from build123d import *

# Parameters (mm, degrees)
SKETCH_1_R          = 13
SKETCH_1_R_2        = 2.6
SKETCH_1_R_3        = 1.4
EXTRUDE_1_DEPTH     = 4
SKETCH_1_3_R        = 13
SKETCH_1_3_R_2      = 2.6
EXTRUDE_2_DEPTH     = 12
EXTRUDE_START       = 11
SKETCH_1_6_R        = 14
SKETCH_1_6_R_2      = 13
EXTRUDE_3_DEPTH     = 1
CUT_EXTRUDE_1_DEPTH = 5
SKETCH_6_R          = 7.6
SKETCH_6_W          = 3
SKETCH_6_H          = 3
CUT_EXTRUDE_5_DEPTH = 5
SKETCH_5_R          = 5
CUT_EXTRUDE_6_DEPTH = 2
FILLET_1_R          = 12
SKETCH_7_R          = 20
SKETCH_7_R_2        = 13
EXTRUDE_5_DEPTH     = 11


with BuildPart() as part:
    # 草图1 → 凸台-拉伸1 (new body)
    # profile 1 of 3: a face of its own
    with BuildSketch(Plane.XY):
        Circle(SKETCH_1_R)
        Circle(SKETCH_1_R_2, mode=Mode.SUBTRACT)
    # profile 2 of 3: a face of its own
    with BuildSketch(Plane.XY):
        with BuildLine():
            Line((-1.6, -2.049390153), (-1.6, 2.049390153))
            ThreePointArc((-1.6, 2.049390153), (-2.6, 0), (-1.6, -2.049390153))
        make_face()
    # profile 3 of 3: a face of its own
    with BuildSketch(Plane.XY):
        with BuildLine():
            ThreePointArc((2.6, 0), (1.140175425, 2.336664289), (-1.6, 2.049390153))
            Line((-1.6, 2.049390153), (-1.6, -2.049390153))
            ThreePointArc((-1.6, -2.049390153), (1.140175425, -2.336664289), (2.6, 0))
        make_face()
        Circle(SKETCH_1_R_3, mode=Mode.SUBTRACT)
    extrude(amount=EXTRUDE_1_DEPTH)

    # 草图1<3> → 凸台-拉伸2 (add)
    # profile 1 of 2: a face of its own
    with BuildSketch(Plane.XY):
        Circle(SKETCH_1_3_R)
        Circle(SKETCH_1_3_R_2, mode=Mode.SUBTRACT)
    # profile 2 of 2: a face of its own
    with BuildSketch(Plane.XY):
        with BuildLine():
            Line((-1.6, -2.049390153), (-1.6, 2.049390153))
            ThreePointArc((-1.6, 2.049390153), (-2.6, 0), (-1.6, -2.049390153))
        make_face()
    extrude(amount=EXTRUDE_2_DEPTH)

    # 草图1<6> → 凸台-拉伸3 (add)
    with BuildSketch(Plane.XY.offset(EXTRUDE_START)):
        Circle(SKETCH_1_6_R)
        Circle(SKETCH_1_6_R_2, mode=Mode.SUBTRACT)
    extrude(amount=EXTRUDE_3_DEPTH)

    # 草图3 → 切除-拉伸1 (cut)
    with BuildSketch(Plane(origin=(0, 0, 0), x_dir=(-1, 0, 0), z_dir=(0, 0, -1))):
        with BuildLine():
            Line((-10.746987514, -5.338750731), (-4.305410284, -1.619704383))
            ThreePointArc((-4.305410284, -1.619704383), (-3.983716857, 2.3), (-0.75, 4.538446871))
            Line((-0.75, 4.538446871), (-0.75, 11.976539567))
            ThreePointArc((-0.75, 11.976539567), (-10.392304845, 6), (-10.746987514, -5.338750731))
        make_face()
        with BuildLine():
            Line((9.996987514, -6.637788836), (3.555410284, -2.918742488))
            ThreePointArc((3.555410284, -2.918742488), (0, -4.6), (-3.555410284, -2.918742488))
            Line((-3.555410284, -2.918742488), (-9.996987514, -6.637788836))
            ThreePointArc((-9.996987514, -6.637788836), (0, -12), (9.996987514, -6.637788836))
        make_face()
        with BuildLine():
            ThreePointArc((4.6, 0), (4.52575338, -0.823138109), (4.305410284, -1.619704383))
            Line((4.305410284, -1.619704383), (10.746987514, -5.338750731))
            ThreePointArc((10.746987514, -5.338750731), (11.682547885, -2.741910814), (12, 0))
            ThreePointArc((12, 0), (8.746427842, 8.215838363), (0.75, 11.976539567))
            Line((0.75, 11.976539567), (0.75, 4.538446871))
            ThreePointArc((0.75, 4.538446871), (3.507848343, 2.975735203), (4.6, 0))
        make_face()
    extrude(amount=-CUT_EXTRUDE_1_DEPTH, mode=Mode.SUBTRACT)

    # 草图6 → 切除-拉伸5 (cut)
    with BuildSketch(Plane.XY.offset(12)):
        Circle(SKETCH_6_R)
        with Locations((-8.950503339, 0)):
            Rectangle(SKETCH_6_W, SKETCH_6_H)
    extrude(amount=-CUT_EXTRUDE_5_DEPTH, mode=Mode.SUBTRACT)

    # 草图5 → 切除-拉伸6 (cut)
    with BuildSketch(Plane(origin=(0, 0, 0), x_dir=(-1, 0, 0), z_dir=(0, 0, -1))):
        Circle(SKETCH_5_R)
    extrude(amount=-CUT_EXTRUDE_6_DEPTH, mode=Mode.SUBTRACT)

    # 圆角1
    # the kernel refuses this fillet: 12 mm, written as the material it takes off along each edge
    with BuildSketch(Plane(origin=(0, 0, 0), x_dir=(-0.0031415874858860904, -0.9999950652018581, 0), z_dir=(0.9999950652018581, -0.0031415874858860904, 0))) as fillet_1_piece_1:
        with BuildLine():
            CenterArc((11.633249581, -12), FILLET_1_R, 90, 33.557309762)
            Line((5, -2), (5, 0))
            Line((5, 0), (11.633249581, 0))
        make_face()
    revolve(axis=Axis((0, 0, 0), (0, 0, -1)), revolution_arc=359.64, mode=Mode.SUBTRACT)
    with BuildSketch(Plane(origin=(0, 0, 0), x_dir=(0.8675919238668026, 0.49727683802998507, 0), z_dir=(-0.49727683802998507, 0.8675919238668026, 0))) as fillet_1_piece_2:
        with BuildLine():
            CenterArc((11.633249581, -12), FILLET_1_R, 90, 33.557309762)
            Line((5, -2), (5, 0))
            Line((5, 0), (11.633249581, 0))
        make_face()
    revolve(axis=Axis((0, 0, 0), (0, 0, -1)), revolution_arc=359.64, mode=Mode.SUBTRACT)
    with BuildSketch(Plane(origin=(0, 0, 0), x_dir=(-0.8644503363809427, 0.5027182271719167, 0), z_dir=(-0.5027182271719167, -0.8644503363809427, 0))) as fillet_1_piece_3:
        with BuildLine():
            CenterArc((11.633249581, -12), FILLET_1_R, 90, 33.557309762)
            Line((5, -2), (5, 0))
            Line((5, 0), (11.633249581, 0))
        make_face()
    revolve(axis=Axis((0, 0, 0), (0, 0, -1)), revolution_arc=359.64, mode=Mode.SUBTRACT)

    # 草图7 → 凸台-拉伸5 (add)
    with BuildSketch(Plane(origin=(0, 0, 11), x_dir=(-1, 0, 0), z_dir=(0, 0, -1)).offset(EXTRUDE_START)):
        with Locations(Location((0, 0, 0), (0, 0, 180))):
            Circle(SKETCH_7_R)
        Circle(SKETCH_7_R_2, mode=Mode.SUBTRACT)
    extrude(amount=-EXTRUDE_5_DEPTH)


solid = part.part
The model under review builds one solid part; all positions refer to its coordinate system, in mm. A direction names the side the tool comes from. Coordinates: 2 decimals unless noted, no trailing zeros. Order: outer loops, then holes, each group sorted by start corner. A loop starts at its lowest first (then second) coordinate and runs counter-clockwise, first axis right, second up. Notation, with made-up numbers: (68, 86.5) -> (92, 86.5) arc R14 ccw to (92, 102.5) -> close; hole circle Ø9 at (62.25, 23.5). An arc over 180 degrees is marked (long way). Answer in a Markdown table with one row per item.
(1) The part is to be moulded in two halves that separate along X. For faces 4 (the cylindrical face through (-19.98, -0.88, 5.42)), 5 (the flat face through (-1.6, 0, 5)), 6 (the flat face through (6, -6, 12)), say which applies: +X half, -X half, draft (parallel to the pull), parting line (faces both ways), or undercut.
Answers:
| item | result |
|---|---|
| face 4 | parting line |
| face 5 | undercut |
| face 6 | draft |
(2) Wall thickness on line 1 along Y through (x, z) = (0, 6.1); line 2 along Y through (x, z) = (0, 9.85); line 3 along Y through (x, z) = (-6.5, 4.75): over which ranges is each line inside the solid? List them lowest first.
Answers:
| item | result |
|---|---|
| line 1 | -20 to -2.6, 2.6 to 20 |
| line 2 | -20 to -7.6, 7.6 to 20 |
| line 3 | -18.91 to -10.09, -4.62 to -2.89, 10.09 to 18.91 |
(3) Insertion check: pin 1 (1.5 mm diameter, centred on x = -9, z = 9, fed in from -Y); pin 2 (1.3 mm diameter, centred on x = 0.5, y = -0.5, fed in from +Z); pin 3 (1 mm diameter, centred on y = -7, z = 4.5, fed in from +X); pin 4 (8 mm diameter, centred on x = 1, y = -0.5, fed in from -Z). Each pin has a flat end and moves straight along its axis. Give the tip position at first contact, or say it passes through.
Answers:
| item | result |
|---|---|
| pin 1 | y = -18.22 |
| pin 2 | through |
| pin 3 | x = 18.91 |
| pin 4 | z = 1.92 |
(4) Consider section A-A (z = 8.75). Write out the cut boundary in (x, y), plus the area to 3 significant figures.
Answers:
| item | result |
|---|---|
| outline | circle Ø40 at (0, 0); hole (-10.45, -1.5) -> (-7.45, -1.5) arc R7.6 ccw (long way) to (-7.45, 1.5) -> (-10.45, 1.5) -> close |
| area | 1,070 mm² |
(5) Consider section B-B (z = 2.5). Write out the cut boundary in (x, y).
Answers:
| item | result |
|---|---|
| outline | circle Ø40 at (0, 0); hole (-10.75, -5.34) -> (-4.31, -1.62) arc R4.6 cw to (-0.75, 4.54) -> (-0.75, 11.98) arc R12 ccw to start; hole (-10, -6.64) arc R12 ccw to (10, -6.64) -> (3.56, -2.92) arc R4.6 cw to (-3.56, -2.92) -> close; hole circle Ø2.8 at (0, 0); hole (0.75, 4.54) arc R4.6 cw to (4.31, -1.62) -> (10.75, -5.34) arc R12 ccw to (0.75, 11.98) -> close |
(6) Machinability: for faces 1 (the flat face through (6, 3, 5)), 2 (the cylindrical face through (-1.4, 0.06, 2.99)), 3 (the flat face through (-9, -1.5, 10)), which of the approach directions +Z, -Z, +X, -X, +Y, -Y give a long, thin tool a straight path to every point of the face, cutting with its end or side? Answer none if there is none.
Answers:
| item | result |
|---|---|
| face 1 | -Z |
| face 2 | +Z, -Z |
| face 3 | +Z |
(7) Consider section C-C (z = 5.5). Write out the cut boundary in (x, y).
Answers:
| item | result |
|---|---|
| outline | circle Ø40 at (0, 0); hole (-1.6, -2.05) arc R2.6 ccw (long way) to (-1.6, 2.05) -> close |
